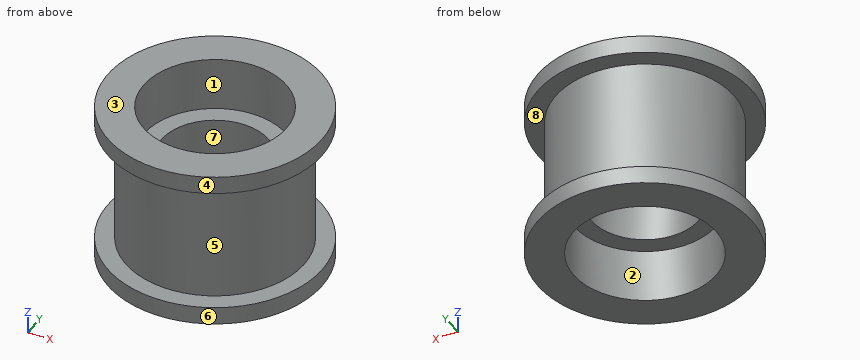
```python
from build123d import *

# Parameters (mm, degrees)
F0_R     = 9.525
F0_R_2   = 4.7625
F1_DEPTH = 14.2875
F2_W     = 1.5875
F2_H     = 11.1125
F4_R     = 6.35
F5_DEPTH = 4.7625
F6_R     = 6.35
F7_DEPTH = 4.7625


with BuildPart() as f1:
    # F0 (on Top) → F1 (new body)
    with BuildSketch(Plane.XY):
        Circle(F0_R)
        Circle(F0_R_2, mode=Mode.SUBTRACT)
    extrude(amount=F1_DEPTH)

    # F2 (on Front) → F3 (revolve, cut)
    with BuildSketch(Plane.XZ):
        with Locations((-8.73125, 7.14375)):
            Rectangle(F2_W, F2_H)
    revolve(axis=Axis((0, 0, 0), (0, 0, -1)), mode=Mode.SUBTRACT)

    # F4 (on face) → F5 (cut)
    with BuildSketch(Plane.XY.offset(14.2875)):
        Circle(F4_R)
    extrude(amount=-F5_DEPTH, mode=Mode.SUBTRACT)

    # F6 (on face) → F7 (cut)
    with BuildSketch(Plane(origin=(0, 0, 0), x_dir=(1, 0, 0), z_dir=(0, 0, -1))):
        Circle(F6_R)
    extrude(amount=-F7_DEPTH, mode=Mode.SUBTRACT)


solid = f1.part
```
Here's how the part is built. I have some questions about the finished solid (model axes, mm). Face numbers are marked on the shaded views. A direction names the side the tool comes from. Coordinates: 2 decimals unless noted, no trailing zeros. Loops run counter-clockwise (first coordinate to the right, second up) from the corner with the lowest first, then second, coordinate; pieces in that order, holes last. Notation, with made-up numbers: (6, 71) - (53, 71) arc R20 cw to (53, 108) - close; hole circle Ø2 at (66.25, 43). An arc over 180 degrees is marked (long way). Answer as CSV lines item,"result".
Q1. For pin 1 (1 mm diameter, centred on y = -4, z = 12, fed in from +X); pin 2 (8 mm diameter, centred on x = 1, y = -1.5, fed in from +Z) (3 decimals); pin 3 (10 mm diameter, centred on x = 0, y = 0, fed in from -Z), each with a flat end and sliding along its axis, tell me the tip position at first contact or that it passes through.
Response:
pin 1,"x = 7.12"
pin 2,"z = 9.525"
pin 3,"z = 4.76"
Q2. If I drill on L1, parallel to Y at x = 0, z = 12; L2, parallel to Y at x = 0, z = 8.1; L3, parallel to Z at x = -3, y = -8, over which ranges is the centre line in solid material (lowest first)? Write a range as [from, to].
Response:
L1,"[-7.94, -6.35], [6.35, 7.94]"
L2,"[-7.94, -4.76], [4.76, 7.94]"
L3,"[0, 1.59], [12.7, 14.29]"
Q3. We'd pull the mould along X, two halves only. Please class the marked faces 6, 7 and 8: pulls with the +X half, pulls with the -X half, needs draft (parallel to the pull), parting line crosses it, or undercut.
Response:
face 6,"parting line crosses it"
face 7,"undercut"
face 8,"needs draft"
Q4. If we section it at C-C, the plane z = 6.5: Write out the boundary of the cut face in (x, y) (1 decimal).
Response:
outline,"circle Ø15.9 at (0, 0); hole circle Ø9.5 at (0, 0)"
Q5. If we section it at D-D, the plane x = 7.25: Write out the boundary of the cut face in (y, z), and give its area (3 significant figures).
Response:
outline,"(-6.18, 0) - (6.18, 0) - (6.18, 1.59) - (3.23, 1.59) - (3.23, 12.7) - (6.18, 12.7) - (6.18, 14.29) - (-6.18, 14.29) - (-6.18, 12.7) - (-3.23, 12.7) - (-3.23, 1.59) - (-6.18, 1.59) - close"
area,"111 mm2"
Q6. For the marked faces 1, 2, 3, 4 and 5, which set-ups out of +Z, -Z, +X, -X, +Y, -Y let a thin tool reach every point of the face, with its end or its side?
Response:
face 1,"+Z"
face 2,"-Z"
face 3,"+Z, +X, -X, +Y, -Y"
face 4,"+Z, -Z"
face 5,"none"
